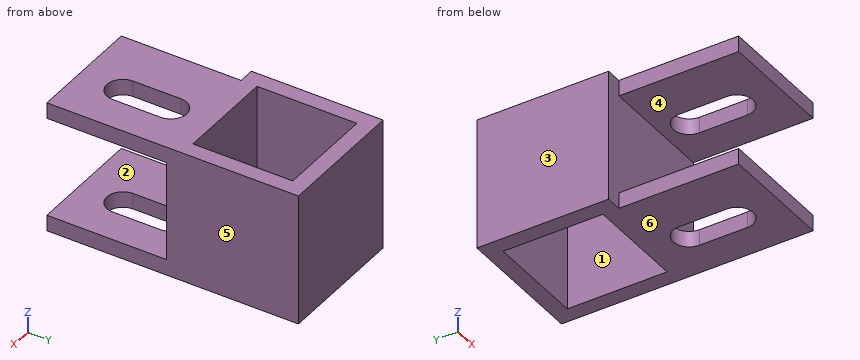
```python
from build123d import *

# Parameters (mm, degrees)
SKETCH20_W                = 33
SKETCH20_H                = 33
SKETCH20_W_2              = 25
SKETCH20_H_2              = 25
BOSS_EXTRUDE12_DEPTH      = 33
BOSS_EXTRUDE13_DEPTH      = 30
BOSS_EXTRUDE13_DEPTH_BACK = 4
SKETCH22_W                = 33
SKETCH22_H                = 4
SKETCH23_W                = 4
SKETCH23_H                = 4
CUT_EXTRUDE10_DEPTH       = 30
CUT_EXTRUDE15_DEPTH       = 33


with BuildPart() as part:
    # Sketch20 → Boss-Extrude12 (new body)
    with BuildSketch(Plane.XY):
        Rectangle(SKETCH20_W, SKETCH20_H)
        Rectangle(SKETCH20_W_2, SKETCH20_H_2, mode=Mode.SUBTRACT)
    extrude(amount=BOSS_EXTRUDE12_DEPTH)

    # Sketch22 → Boss-Extrude13 (add, two sides: drawn at the far end of the back side and taken through both)
    with BuildSketch(Plane.XZ.offset(16.5).offset(-BOSS_EXTRUDE13_DEPTH_BACK)):
        with Locations((0, 31)):
            Rectangle(SKETCH22_W, SKETCH22_H)
        with Locations((0, 2)):
            Rectangle(SKETCH22_W, SKETCH22_H)
    extrude(amount=BOSS_EXTRUDE13_DEPTH + BOSS_EXTRUDE13_DEPTH_BACK)

    # Sketch23 → Cut-Extrude10 (cut)
    with BuildSketch(Plane.XZ.offset(46.5)):
        with Locations((-14.5, 31)):
            Rectangle(SKETCH23_W, SKETCH23_H)
        with Locations((-14.5, 2)):
            Rectangle(SKETCH23_W, SKETCH23_H)
    extrude(amount=-CUT_EXTRUDE10_DEPTH, mode=Mode.SUBTRACT)

    # Sketch36 → Cut-Extrude15 (cut)
    with BuildSketch(Plane(origin=(0, 0, 0), x_dir=(-1, 0, 0), z_dir=(0, 0, -1))):
        with BuildLine():
            Line((-8, -23.5), (-8, -35.5))
            ThreePointArc((-8, -35.5), (-4, -39.5), (0, -35.5))
            Line((0, -35.5), (0, -23.5))
            ThreePointArc((0, -23.5), (-4, -19.5), (-8, -23.5))
        make_face()
    extrude(amount=-CUT_EXTRUDE15_DEPTH, mode=Mode.SUBTRACT)


solid = part.part
```
Input: part model. Units: mm. Frame: model coordinates. Face numbers are marked on the shaded views. A direction names the side the tool comes from. Coordinates: 2 decimals unless noted, no trailing zeros. Loops run counter-clockwise (first coordinate to the right, second up) from the corner with the lowest first, then second, coordinate; pieces in that order, holes last. Notation, with made-up numbers: (43, 47) -> (64, 47) arc R23 ccw to (64, 68) -> close; hole circle Ø9 at (45.25, -34). An arc over 180 degrees is marked (long way). Use a Markdown table: item, result.
1) Cut plane C-C (z = 30.5). Return the cut outline in (x, y).
Results found:
| item | result |
|---|---|
| outline | (-16.5, -16.5) -> (-12.5, -16.5) -> (-12.5, -46.5) -> (16.5, -46.5) -> (16.5, 16.5) -> (-16.5, 16.5) -> close; hole (-12.5, -12.5) -> (12.5, -12.5) -> (12.5, 12.5) -> (-12.5, 12.5) -> close; hole (0, -35.5) arc R4 ccw to (8, -35.5) -> (8, -23.5) arc R4 ccw to (0, -23.5) -> close |
2) Cut plane D-D (y = -25.5). Return the cut outline in (x, z).
Results found:
| item | result |
|---|---|
| outline | (-12.5, 0) -> (0, 0) -> (0, 4) -> (-12.5, 4) -> close; (-12.5, 29) -> (0, 29) -> (0, 33) -> (-12.5, 33) -> close; (8, 0) -> (16.5, 0) -> (16.5, 4) -> (8, 4) -> close; (8, 29) -> (16.5, 29) -> (16.5, 33) -> (8, 33) -> close |
3) Contact query for flat-ended pins moving along their axis: pin 1 (16.5 mm diameter, centred on x = 6, z = 15, fed in from -Y); pin 2 (4.5 mm diameter, centred on y = -38.5, z = 30.5, fed in from -X). Output: stop coordinate, or through.
Results found:
| item | result |
|---|---|
| pin 1 | stops at y = -16.5 |
| pin 2 | stops at x = -12.5 |
4) Access query for the marked faces 1, 2 and 3. Directions: +Z, -Z, +X, -X, +Y, -Y. A direction counts if a zero-diameter tool reaches every point of the face in a straight line with its end or side. Return the directions, or none.
Results found:
| item | result |
|---|---|
| face 1 | +Z, -Z |
| face 2 | +X, -X, -Y |
| face 3 | +Z, -Z, -X, +Y, -Y |
5) Pull-direction query (Z, two-part tool) for the marked faces 4, 5 and 6; classes: released by +Z, released by -Z, zero draft, split by the parting line, or undercut.
Results found:
| item | result |
|---|---|
| face 4 | undercut |
| face 5 | zero draft |
| face 6 | released by -Z |
6) Cut plane A-A (y = 4). Return the cut outline in (x, z).
Results found:
| item | result |
|---|---|
| outline | (-16.5, 0) -> (-12.5, 0) -> (-12.5, 33) -> (-16.5, 33) -> close; (12.5, 0) -> (16.5, 0) -> (16.5, 33) -> (12.5, 33) -> close |
7) Cut plane B-B (x = 4). Return the cut outline in (y, z), then the cut area to 3 significant figures.
Results found:
| item | result |
|---|---|
| outline | (-46.5, 0) -> (-39.5, 0) -> (-39.5, 4) -> (-46.5, 4) -> close; (-46.5, 29) -> (-39.5, 29) -> (-39.5, 33) -> (-46.5, 33) -> close; (-19.5, 0) -> (-12.5, 0) -> (-12.5, 33) -> (-19.5, 33) -> (-19.5, 29) -> (-16.5, 29) -> (-16.5, 4) -> (-19.5, 4) -> close; (12.5, 0) -> (16.5, 0) -> (16.5, 33) -> (12.5, 33) -> close |
| area | 344 mm2 |
8) Material intervals for line 1 along Y through (x, z) = (3.5, 13.5); line 2 along Z through (x, y) = (-10, -27.5), sorted ascending. Write a range as from..to.
Results found:
| item | result |
|---|---|
| line 1 | y = -16.5..-12.5, 12.5..16.5 |
| line 2 | z = 0..4, 29..33 |
